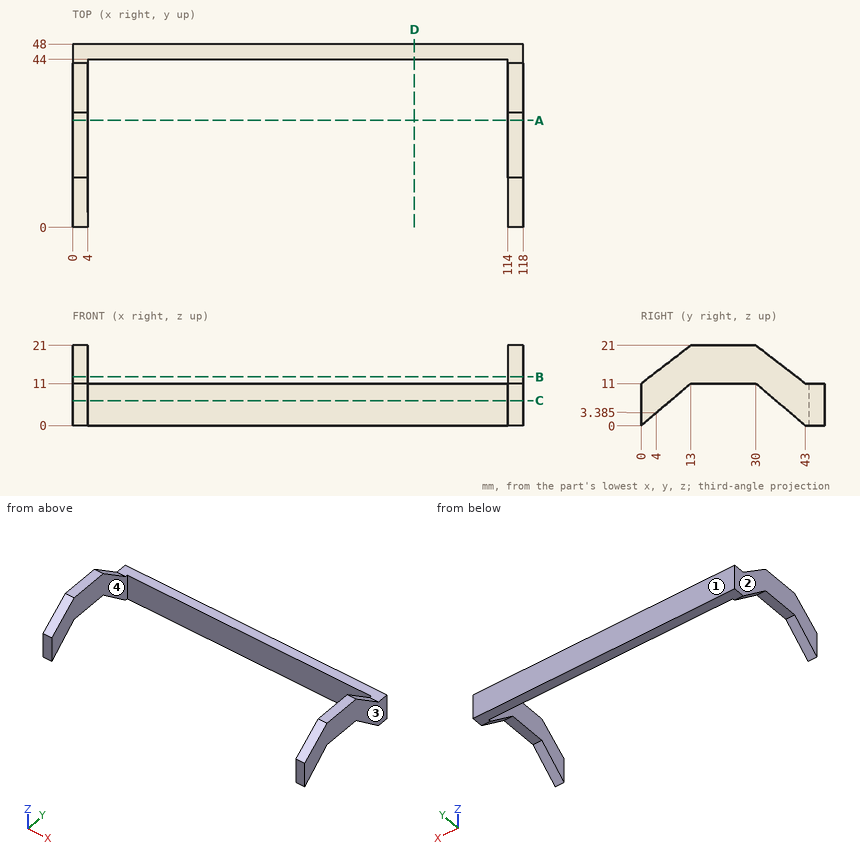
The drawing under review shows one solid part. Ordinate dimensions are in mm from its lowest x, y, z. Coordinates: 2 decimals unless noted, no trailing zeros. Write each loop counter-clockwise with the first axis right and the second up, starting at its lowest first coordinate (ties: lowest second). Pieces come first, ordered by that corner, then holes.
1) Add section D-D (x = 89.5). Write out the cut boundary in (y, z), plus the area to 3 significant figures.
2) Mouldability with a two-part tool opening along X and no side actions: class the marked faces 1, 2, 3 and 4 as +X half, -X half, draft (parallel to the pull), parting line (faces both ways), or undercut.
3) Add section C-C (z = 6.5). Write out the cut boundary in (x, y), plus the area to 3 significant figures.
4) Add section A-A (y = 28). Write out the cut boundary in (x, z), plus the area to 3 significant figures.
5) Insertion check: pin 1 (1.5 mm diameter, centred on x = 77.5, y = 46.5, fed in from +Z); pin 2 (1.5 mm diameter, centred on x = 38, z = 10.5, fed in from -Y); pin 3 (2 mm diameter, centred on x = 115, y = 22, fed in from -Z); pin 4 (10 mm diameter, centred on y = 18.5, z = 3, fed in from +X). Each pin has a flat end and moves straight along its axis. Give the tip position at first contact, or say it passes through.
6) To check wall thickness, follow L1, parallel to X at y = 15.5, z = 16.5; L2, parallel to Y at x = 15.5, z = 1.5; L3, parallel to Z at x = 107, y = 45. State the ranges of each line that lie inside material, in increasing order.
7) Add section B-B (z = 12.75). Write out the cut boundary in (x, y) (1 decimal).
Check result:
1. outline: (44, 0) - (48, 0) - (48, 11) - (44, 11) - close
1. area: 44.0 mm2
2. face 1: draft
2. face 2: -X half
2. face 3: +X half
2. face 4: undercut
3. outline: (0, 0) - (4, 0) - (4, 7.68) - (0, 7.68) - close; (0, 35.32) - (4, 35.32) - (4, 44) - (114, 44) - (114, 35.32) - (118, 35.32) - (118, 48) - (0, 48) - close; (114, 0) - (118, 0) - (118, 7.68) - (114, 7.68) - close
3. area: 603 mm2
4. outline: (0, 11) - (4, 11) - (4, 21) - (0, 21) - close; (114, 11) - (118, 11) - (118, 21) - (114, 21) - close
4. area: 80.0 mm2
5. pin 1: stops at z = 11
5. pin 2: stops at y = 44
5. pin 3: stops at z = 11
5. pin 4: passes through
6. L1: x = 0 to 4, 114 to 118
6. L2: y = 44 to 48
6. L3: z = 0 to 11
7. outline: (0, 2.3) - (4, 2.3) - (4, 40.7) - (0, 40.7) - close; (114, 2.3) - (118, 2.3) - (118, 40.7) - (114, 40.7) - close
